Could you check a few things on this model? Use its own coordinates, in mm. A direction names the side the tool comes from. Coordinates: 2 decimals unless noted, no trailing zeros. Order: outer loops, then holes, each group sorted by start corner. A loop starts at its lowest first (then second) coordinate and runs counter-clockwise, first axis right, second up. Notation, with made-up numbers: (42, 83.25) -> (81, 83.25) arc R20 ccw to (81, 114.25) -> close; hole circle Ø9 at (33, 50.5). An arc over 180 degrees is marked (long way). Use a Markdown table: item, result. Add a question column.
1) Thinking about a two-plate mould opening in Y: for faces 6 (the flat face through (-5, 3, 3)), 7 (the flat face through (-9, 10.5, 1)), 8 (the cylindrical face through (5.811, -10.275, 1.521)), which applies, +Y half, -Y half, draft (parallel to the pull), parting line (faces both ways), or undercut?
2) If we section it at D-D (x = -6.5): Write out the boundary of the cut face in (y, z), plus the area to 3 significant figures.
3) If we section it at C-C (y = -1): Write out the boundary of the cut face in (x, z).
4) Will these pins go through, and if not, where does the flat tip stop? pin 1 Ø1.3 at (y, z) = (-12.5, 2) entering from +X; pin 2 Ø0.8 at (y, z) = (12.5, 2) entering from -X; pin 3 Ø1.5 at (x, z) = (9, 2) entering from -Y.
5) If I drill on L1, parallel to X at y = -11, z = 1.1; L2, parallel to Y at x = 6.5, z = 1.55; L3, parallel to Y at x = 0, z = 2.1, over which ranges is the centre line in solid material (lowest first)? Write a range as [from, to].
6) Which directions (+Z, -Z, +X, -X, +Y, -Y) give clear straight access to the entire face, cutting with the end or side of a thin tool? Please do faces 1 (the cylindrical face through (-5.811, 10.275, 1.521)), 2 (the flat face through (-6, 13, 1)), 3 (the flat face through (-6, -13, 1)), 4 (the flat face through (6, 13, 1)), 5 (the flat face through (9, -10.5, 1)).
7) If we section it at A-A (x = 0): Write out the boundary of the cut face in (y, z), plus the area to 3 significant figures.
8) If we section it at B-B (z = 2.7): Write out the boundary of the cut face in (x, y), plus the area to 3 significant figures.
```python
from build123d import *

# Parameters (mm, degrees)
SKETCH_1_W          = 12
SKETCH_1_H          = 3
SKETCH_1_H_2        = 21
SKETCH_1_W_2        = 4.5
EXTRUDE_1_DEPTH     = 3
SKETCH_2_R          = 5
CUT_EXTRUDE_1_DEPTH = 18.363755354
SKETCH_3_R          = 1
CUT_EXTRUDE_2_DEPTH = 18.363755354


with BuildPart() as part:
    # 草图1 → 凸台-拉伸1 (new body)
    with BuildSketch(Plane.XY):
        with Locations((0, 12)):
            Rectangle(SKETCH_1_W, SKETCH_1_H)
        Rectangle(SKETCH_1_W, SKETCH_1_H_2)
        with Locations((8.25, 0)):
            Rectangle(SKETCH_1_W_2, SKETCH_1_H_2)
        with Locations((0, -12)):
            Rectangle(SKETCH_1_W, SKETCH_1_H)
        with Locations((-8.25, 0)):
            Rectangle(SKETCH_1_W_2, SKETCH_1_H_2)
    extrude(amount=EXTRUDE_1_DEPTH)

    # 草图2 → 切除-拉伸1 (cut, through all)
    with BuildSketch(Plane.XY.offset(3)):
        Circle(SKETCH_2_R)
    extrude(amount=-CUT_EXTRUDE_1_DEPTH, mode=Mode.SUBTRACT)

    # 草图3 → 切除-拉伸2 (cut, through all)
    with BuildSketch(Plane.XY.offset(3)):
        with Locations((-6.5, 11)):
            Circle(SKETCH_3_R)
        with Locations((6.5, 11)):
            Circle(SKETCH_3_R)
        with Locations((6.5, -11)):
            Circle(SKETCH_3_R)
        with Locations((-6.5, -11)):
            Circle(SKETCH_3_R)
    extrude(amount=-CUT_EXTRUDE_2_DEPTH, mode=Mode.SUBTRACT)


solid = part.part
```
Answer sheet:
| question | item | result |
|---|---|---|
| 1 | face 6 | draft |
| 1 | face 7 | +Y half |
| 1 | face 8 | undercut |
| 2 | outline | (-10, 0) -> (10, 0) -> (10, 3) -> (-10, 3) -> close |
| 2 | area | 60.0 mm2 |
| 3 | outline | (-10.5, 0) -> (-4.9, 0) -> (-4.9, 3) -> (-10.5, 3) -> close; (4.9, 0) -> (10.5, 0) -> (10.5, 3) -> (4.9, 3) -> close |
| 4 | pin 1 | x = 6 |
| 4 | pin 2 | x = -6 |
| 4 | pin 3 | y = -10.5 |
| 5 | L1 | [-5.5, 5.5] |
| 5 | L2 | [-10, 10] |
| 5 | L3 | [-13.5, -5], [5, 13.5] |
| 6 | face 1 | +Z, -Z |
| 6 | face 2 | +Z, -Z, -X, +Y |
| 6 | face 3 | +Z, -Z, -X, -Y |
| 6 | face 4 | +Z, -Z, +X, +Y |
| 6 | face 5 | +Z, -Z, +X, -Y |
| 7 | outline | (-13.5, 0) -> (-5, 0) -> (-5, 3) -> (-13.5, 3) -> close; (5, 0) -> (13.5, 0) -> (13.5, 3) -> (5, 3) -> close |
| 7 | area | 51.0 mm2 |
| 8 | outline | (-10.5, -10.5) -> (-7.37, -10.5) arc R1 cw (long way) to (-6, -11.87) -> (-6, -13.5) -> (6, -13.5) -> (6, -11.87) arc R1 cw (long way) to (7.37, -10.5) -> (10.5, -10.5) -> (10.5, 10.5) -> (7.37, 10.5) arc R1 cw (long way) to (6, 11.87) -> (6, 13.5) -> (-6, 13.5) -> (-6, 11.87) arc R1 cw (long way) to (-7.37, 10.5) -> (-10.5, 10.5) -> close; hole circle Ø10 at (0, 0) |
| 8 | area | 430 mm2 |
